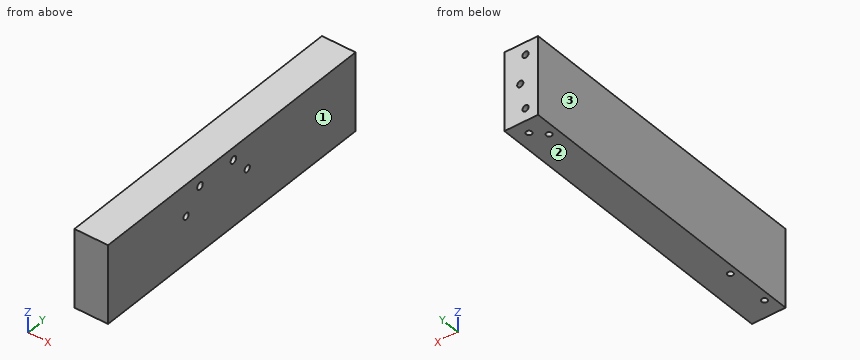
Autodesk Inventor part; units mm, degrees
ref_plane "YZ Plane" through (0, 0, 0) normal (1, 0, 0) x (0, 1, 0)
ref_plane "XZ Plane" through (0, 0, 0) normal (0, 1, 0) x (-1, 0, 0)
ref_plane "XY Plane" through (0, 0, 0) normal (0, 0, 1) x (1, 0, 0)
sketch "Sketch1" plane through (0, 0, 0) normal (0, 1, 0) x (-1, 0, 0)
  line L0 (0, 0) -> (-38.1, 0)
  line L1 (-38.1, 0) -> (-38.1, -88.9)
  line L2 (-38.1, -88.9) -> (0, -88.9)
  line L3 (0, -88.9) -> (0, 0)
  dimension "d0" = 38.1
  dimension "d1" = 88.9
extrude "Extrusion1" add sketch "Sketch1" along normal blind 355.6
sketch "Sketch3" plane through (0, 355.6, 0) normal (0, 1, 0) x (1, 0, 0)
  line L0 (14.2, 74.725) -> (14.2, 14.175)
  line L1 (38.1, 88.9) -> (0, 88.9)
  line L2 (0, 0) -> (38.1, 0)
  line L3 (14.2, 44.45) -> (20.2, 44.45)
  line L4 (0, 88.9) -> (0, 0)
  dimension "d59" = 60.55
  dimension "d60" = 14.175
  dimension "d61" = 14.175
  dimension "d62" = 6
  dimension "d63" = 30.275
  dimension "d64" = 20.2
hole "Hole1" at (14.2, 355.6, -74.725) at (20.2, 355.6, -44.45) at (14.2, 355.6, -14.175) direction (0, -1, 0) diameter 7 depth 10 tip angle 118
sketch "Sketch5" plane through (38.1, 0, -88.9) normal (0, 0, -1) x (-1, 0, 0)
  line L0 (0, 355.6) -> (28.2843, 327.3157)
  line L1 (0, 355.6) -> (38.1, 355.6)
  circle A0 centre (28.2843, 327.3157) radius 2.35
  circle A1 centre (15.5563, 340.0437) radius 2.35
  point P0 (38.1, 0)
  dimension "d25" = 45
  dimension "d26" = 40
  dimension "d27" = 4.7
  dimension "d28" = 4.7
  dimension "d29" = 18
hole "Hole2" at (9.8157, 327.3157, -88.9) at (22.5437, 340.0437, -88.9) direction (0, 0, 1) diameter 6.5 depth 10
sketch "Sketch6" plane through (38.1, 0, -88.9) normal (0, 0, -1) x (-1, 0, 0)
  line L0 (0, 0) -> (0, 355.6)
  line L1 (0, 0) -> (30, 0)
  line L2 (30, 0) -> (30, 20)
  line L3 (30, 20) -> (0, 20)
  line L4 (0, 20) -> (0, 0)
  line L5 (30, 20) -> (30, 68.9)
  circle A0 centre (30, 20) radius 6.1957
  circle A1 centre (30, 68.9) radius 5.1366
  point P0 (38.1, 0)
  dimension "d37" = 30
  dimension "d38" = 20
  dimension "d39" = 48.9
hole "Hole3" at (8.1, 20, -88.9) at (8.1, 68.9, -88.9) direction (0, 0, 1) diameter 6.5 depth 10
sketch "Sketch7" plane through (38.1, 0, 0) normal (1, 0, 0) x (0, 0, -1)
  line L0 (0, 0) -> (36, 0)
  line L1 (36, 0) -> (36, 200)
  line L2 (36, 200) -> (0, 200)
  line L3 (0, 200) -> (0, 0)
  circle A0 centre (36, 200) radius 3.75
  circle A1 centre (36, 112.15) radius 3.75
  dimension "d47" = 36
  dimension "d48" = 200
  dimension "d49" = 87.85
  dimension "d50" = 7.5
  dimension "d51" = 7.5
  dimension "d65" = 112.15
hole "Hole4" at (38.1, 112.15, -36) at (38.1, 200, -36) direction (-1, 0, 0) diameter 7.5 depth 10
sketch "Sketch8" plane through (38.1, 0, 0) normal (1, 0, 0) x (0, 0, -1)
  line L0 (0, 0) -> (14, 0)
  line L1 (14, 0) -> (14, 156.083) construction
  line L2 (14, 156.083) -> (0, 156.083)
  line L3 (0, 156.083) -> (0, 0)
  line L4 (14, 156.083) -> (14, 132.083)
  line L5 (14, 156.083) -> (14, 180.083)
  circle A0 centre (14, 132.083) radius 4
  circle A1 centre (14, 180.083) radius 4
  dimension "d66" = 156.083
  dimension "d67" = 14
  dimension "d69" = 24
  dimension "d70" = 24
  dimension "d71" = 8
  dimension "d72" = 8
extrude "Extrusion2" cut sketch "Sketch8" against normal blind 10
properties part number "thigh2x4" material "Wood (Birch)"
Read the model definition and answer for the solid it produces. Units are mm, in the model's axes. Face numbers are marked on the shaded views. Give positions to 0.01 mm unless a question says otherwise; leave off trailing zeros. Write each loop counter-clockwise with the first axis right and the second up, starting at its lowest first coordinate (ties: lowest second). Pieces come first, ordered by that corner, then holes. Notation, with made-up numbers: (-21, 86) - (5, 86) arc R19 cw to (5, 95) - close; hole circle Ø11 at (9, -13). An arc over 180 degrees is marked (long way). Write item = value, one per line. Start each with the question number.
Item 1: Find section A-A (y = 112.15). Give the vertices of the cut face in (x, z), then the cut area to 3 significant figures.
Item 2: Find section B-B (y = 20). Give the vertices of the cut face in (x, z).
Item 3: Find the intervals of material crossed by probe 1 along Z at (x, y) = (14.2, 353.75) (3 decimals); probe 2 along Y at (x, z) = (31, -36); probe 3 along Z at (x, y) = (20.2, 351.5), in increasing order. Write a range as [from, to].
Item 4: This flat-tipped pin is pushed along its axis until it touches: P1, Ø6, axis at x = 8.1, y = 68.9, coming from the -Z side. Where does it stop, or does it pass through?
Item 5: The mould has two halves that part along X. Classify the marked faces 1, 2 and 3: +X half, -X half, draft (parallel to the pull), parting line (faces both ways), or undercut.
Response:
q1.outline = (0, -88.9) - (38.1, -88.9) - (38.1, -39.75) - (28.1, -39.75) - (28.1, -32.25) - (38.1, -32.25) - (38.1, 0) - (0, 0) - close
q1.area = 3,310 mm²
q2.outline = (0, -88.9) - (4.85, -88.9) - (4.85, -78.9) - (11.35, -78.9) - (11.35, -88.9) - (38.1, -88.9) - (38.1, 0) - (0, 0) - close
q3.probe_1 = [-88.9, -78.225], [-71.225, -17.675], [-10.675, 0]
q3.probe_2 = [0, 108.4], [115.9, 196.25], [203.75, 355.6]
q3.probe_3 = [-88.9, -47.95], [-40.95, 0]
q4.P1 = -78.9
q5.face_1 = +X half
q5.face_2 = draft
q5.face_3 = -X half
